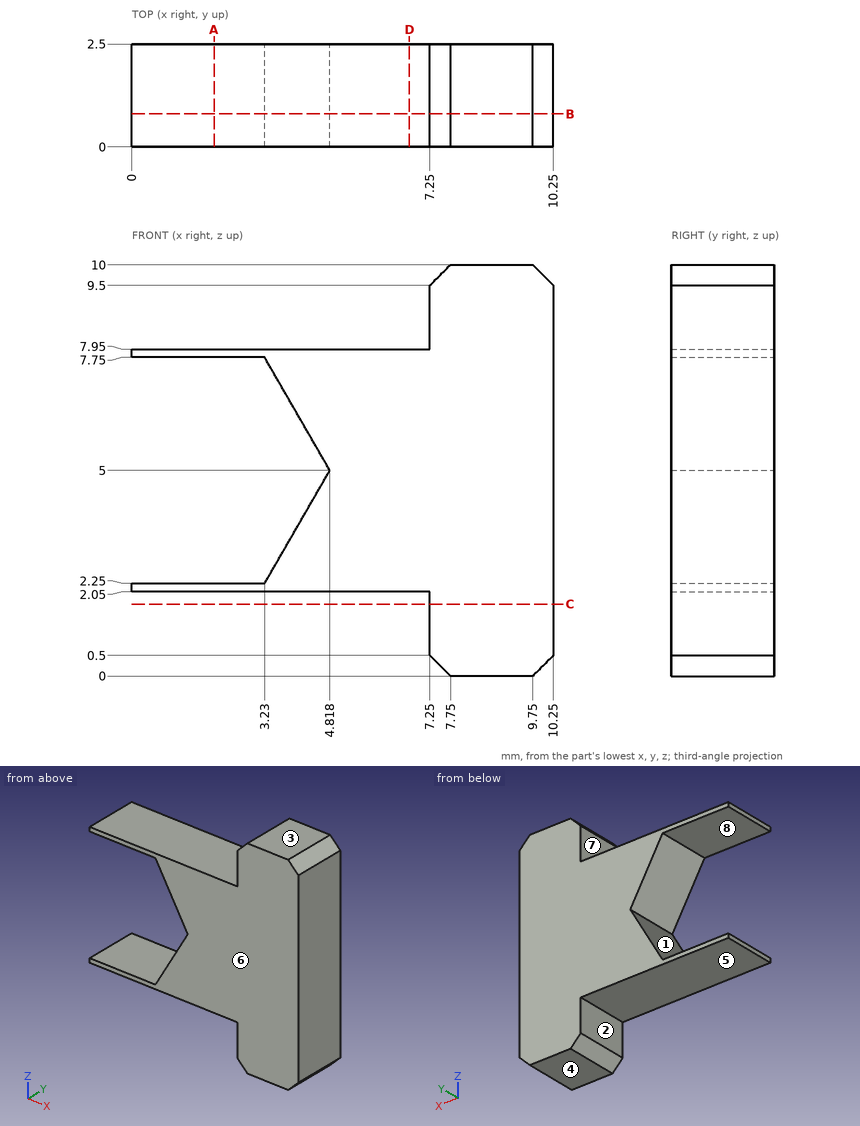
Check sheet for the drawn part. Datum: minimum x, y, z corner. Units: mm. A direction names the side the tool comes from. Give positions to 0.01 mm unless a question says otherwise; leave off trailing zeros. Order: outer loops, then holes, each group sorted by start corner. A loop starts at its lowest first (then second) coordinate and runs counter-clockwise, first axis right, second up. Notation, with made-up numbers: (-36.5, 33) - (18.5, 33) arc R30 cw to (18.5, 67) - close; hole circle Ø9 at (-39, -29.5). An arc over 180 degrees is marked (long way). Answer in a Markdown table with one row per item. Add a question column.
Q1. Cross-section at C-C, the plane z = 1.75. Enter the section's corners in (x, y).
Q2. Cross-section at B-B, the plane y = 0.8. Enter the section's corners in (x, z).
Q3. Tool access check on the marked faces 4, 5, 6, 7 and 8. Record the directions out of +Z, -Z, +X, -X, +Y, -Y that give a thin tool (end or side, any length) a straight path to the whole face; none if there is none.
Q4. Mould release check, pull along Z, two halves, no side actions. Record for the marked faces 1, 2 and 3: pulls with the +Z half, pulls with the -Z half, needs draft (parallel to the pull), parting line crosses it, or undercut.
Q5. Cross-section at D-D, the plane x = 6.75. Enter the section's corners in (y, z).
Q6. Cross-section at A-A, the plane x = 2. Enter the section's corners in (y, z).
Q7. Gauge pin test, flat ends, axial feed: pin 1 (0.8 mm diameter, centred on x = 4.5, y = 1.5, fed in from +Z); pin 2 (0.8 mm diameter, centred on x = 3.5, y = 1, fed in from -Z). Record the tip position at first contact, or that the pin passes through.
Q8. Material ranges on probe 1 along Z at (x, y) = (1.75, 1.4); probe 2 along Z at (x, y) = (6.25, 1.3); probe 3 along X at (y, z) = (0.55, 8.5), recorded low to high. Write a range as from..to.
Check values:
| question | item | result |
|---|---|---|
| 1 | outline | (7.25, 0) - (10.25, 0) - (10.25, 2.5) - (7.25, 2.5) - close |
| 2 | outline | (0, 2.05) - (7.25, 2.05) - (7.25, 0.5) - (7.75, 0) - (9.75, 0) - (10.25, 0.5) - (10.25, 9.5) - (9.75, 10) - (7.75, 10) - (7.25, 9.5) - (7.25, 7.95) - (0, 7.95) - (0, 7.75) - (3.23, 7.75) - (4.82, 5) - (3.23, 2.25) - (0, 2.25) - close |
| 3 | face 4 | -Z, +X, -X, +Y, -Y |
| 3 | face 5 | -Z, -X, +Y, -Y |
| 3 | face 6 | +Z, -Z, +X, -X, -Y |
| 3 | face 7 | +Z, -X, +Y, -Y |
| 3 | face 8 | -X, +Y, -Y |
| 4 | face 1 | undercut |
| 4 | face 2 | needs draft |
| 4 | face 3 | pulls with the +Z half |
| 5 | outline | (0, 2.05) - (2.5, 2.05) - (2.5, 7.95) - (0, 7.95) - close |
| 6 | outline | (0, 2.05) - (2.5, 2.05) - (2.5, 2.25) - (0, 2.25) - close; (0, 7.75) - (2.5, 7.75) - (2.5, 7.95) - (0, 7.95) - close |
| 7 | pin 1 | stops at z = 7.95 |
| 7 | pin 2 | stops at z = 2.05 |
| 8 | probe 1 | z = 2.05..2.25, 7.75..7.95 |
| 8 | probe 2 | z = 2.05..7.95 |
| 8 | probe 3 | x = 7.25..10.25 |
